```python
from build123d import *

# Parameters (mm, degrees)
SKETCH2_R           = 10.5
SKETCH2_R_2         = 7.5
BOSS_EXTRUDE1_DEPTH = 2.5
SKETCH2_3_R         = 7.5
SKETCH2_3_R_2       = 6.5
BOSS_EXTRUDE2_DEPTH = 1.5
SKETCH3_W           = 30
SKETCH3_H           = 6
CUT_EXTRUDE1_DEPTH  = 0.5
CUT_EXTRUDE2_START  = -1.5
CUT_EXTRUDE2_DEPTH  = 1.5
SKETCH5_R           = 5
SKETCH5_R_2         = 3.65
BOSS_EXTRUDE3_DEPTH = 1.5
FILLET1_R           = 0.5
CUT_EXTRUDE3_START  = -2.5
CUT_EXTRUDE3_DEPTH  = 2.5
BOSS_EXTRUDE4_DEPTH = 1.5
FILLET2_R           = 0.2


# Read off the part's stored shape, not the designer's step: Cut-Extrude3
with BuildPart() as part:
    # Sketch2 → Boss-Extrude1 (new body)
    with BuildSketch(Plane(origin=(0, 0, 0), x_dir=(1, 0, 0), z_dir=(0, 1, 0))):
        with Locations(Location((0, 0, 0), (0, 0, 270))):
            Circle(SKETCH2_R)
        with Locations(Location((0, 0, 0), (0, 0, 270))):
            Circle(SKETCH2_R_2, mode=Mode.SUBTRACT)
    extrude(amount=BOSS_EXTRUDE1_DEPTH)

    # Sketch2<3> → Boss-Extrude2 (add)
    with BuildSketch(Plane(origin=(0, 0, 0), x_dir=(1, 0, 0), z_dir=(0, 1, 0))):
        with Locations(Location((0, 0, 0), (0, 0, 270))):
            Circle(SKETCH2_3_R)
        with Locations(Location((0, 0, 0), (0, 0, 270))):
            Circle(SKETCH2_3_R_2, mode=Mode.SUBTRACT)
    extrude(amount=BOSS_EXTRUDE2_DEPTH)

    # Sketch3 → Cut-Extrude1 (cut)
    with BuildSketch(Plane(origin=(0, 2.5, 0), x_dir=(1, 0, 0), z_dir=(0, 1, 0))):
        Rectangle(SKETCH3_W, SKETCH3_H)
    extrude(amount=-CUT_EXTRUDE1_DEPTH, mode=Mode.SUBTRACT)

    # Sketch4 → Cut-Extrude2 (cut)
    with BuildSketch(Plane(origin=(0, 2.5, 0), x_dir=(1, 0, 0), z_dir=(0, 1, 0)).offset(CUT_EXTRUDE2_START)):
        with BuildLine():
            Line((-4, -9.708243919), (4, -9.708243919))
            ThreePointArc((4, -9.708243919), (0, -8.05), (-4, -9.708243919))
        make_face()
        with BuildLine():
            ThreePointArc((-4, -9.708243919), (0, -10.5), (4, -9.708243919))
            Line((4, -9.708243919), (-4, -9.708243919))
        make_face()
    extrude(amount=CUT_EXTRUDE2_DEPTH, mode=Mode.SUBTRACT)

    # Sketch5 → Boss-Extrude3 (add)
    # profile 1 of 6: a face of its own
    with BuildSketch(Plane(origin=(0, 0, 0), x_dir=(1, 0, 0), z_dir=(0, 1, 0))):
        Circle(SKETCH5_R)
        Circle(SKETCH5_R_2, mode=Mode.SUBTRACT)
    # profile 2 of 6: a face of its own
    with BuildSketch(Plane(origin=(0, 0, 0), x_dir=(1, 0, 0), z_dir=(0, 1, 0))):
        with BuildLine():
            Line((-4.307149461, -2.539382508), (-5.394288115, -3.626521162))
            ThreePointArc((-5.394288115, -3.626521162), (-4.596194078, -4.596194078), (-3.626521162, -5.394288115))
            Line((-3.626521162, -5.394288115), (-2.539382508, -4.307149461))
            ThreePointArc((-2.539382508, -4.307149461), (-3.535533906, -3.535533906), (-4.307149461, -2.539382508))
        make_face()
    # profile 3 of 6: a face of its own
    with BuildSketch(Plane(origin=(0, 0, 0), x_dir=(1, 0, 0), z_dir=(0, 1, 0))):
        with BuildLine():
            ThreePointArc((2.965697363, -2.127707487), (3.308023423, -1.542556655), (3.536232016, -0.904191975))
            Line((3.536232016, -0.904191975), (2.777613741, -0.550442464))
            Line((2.777613741, -0.550442464), (2.207079088, -1.773957976))
            Line((2.207079088, -1.773957976), (2.965697363, -2.127707487))
        make_face()
    # profile 4 of 6: a face of its own
    with BuildSketch(Plane(origin=(0, 0, 0), x_dir=(1, 0, 0), z_dir=(0, 1, 0))):
        with BuildLine():
            Line((-2.639832216, -1.02440757), (-3.325497417, -1.504515512))
            ThreePointArc((-3.325497417, -1.504515512), (-2.989904962, -2.093553993), (-2.551169228, -2.610370772))
            Line((-2.551169228, -2.610370772), (-1.865504027, -2.13026283))
            Line((-1.865504027, -2.13026283), (-2.639832216, -1.02440757))
        make_face()
    # profile 5 of 6: a face of its own
    with BuildSketch(Plane(origin=(0, 0, 0), x_dir=(1, 0, 0), z_dir=(0, 1, 0))):
        with BuildLine():
            Line((0.432753129, 2.798365546), (0.359800054, 3.632223))
            ThreePointArc((0.359800054, 3.632223), (-0.318118461, 3.636110648), (-0.985062788, 3.514562747))
            Line((-0.985062788, 3.514562747), (-0.912109714, 2.680705293))
            Line((-0.912109714, 2.680705293), (0.432753129, 2.798365546))
        make_face()
    # profile 6 of 6: a face of its own
    with BuildSketch(Plane(origin=(0, 0, 0), x_dir=(1, 0, 0), z_dir=(0, 1, 0))):
        with BuildLine():
            ThreePointArc((5.394288115, 3.626521162), (4.596194078, 4.596194078), (3.626521162, 5.394288115))
            Line((3.626521162, 5.394288115), (2.539382508, 4.307149461))
            ThreePointArc((2.539382508, 4.307149461), (3.535533906, 3.535533906), (4.307149461, 2.539382508))
            Line((4.307149461, 2.539382508), (5.394288115, 3.626521162))
        make_face()
    extrude(amount=BOSS_EXTRUDE3_DEPTH)

    # Fillet1
    fillet1_edges = [part.edges().sort_by_distance(p)[0] for p in [
        (5.394288115, 0.75, -3.626521162),
        (3.626521162, 0.75, -5.394288115),
        (-5.394288115, 0.75, 3.626521162),
        (-3.626521162, 0.75, 5.394288115),
    ]]
    fillet(fillet1_edges, radius=FILLET1_R)

    # Cut-Extrude3 outline → Cut-Extrude3 (cut)
    with BuildSketch(Plane(origin=(0, 2.5, 0), x_dir=(1, 0, 0), z_dir=(0, 1, 0)).offset(CUT_EXTRUDE3_START)):
        with BuildLine():
            Line((-1.104124308, 7.273205617), (-0.895875692, 6.437966041))
            ThreePointArc((-0.895875692, 6.437966041), (0, 6.5), (0.895875692, 6.437966041))
            Line((0.895875692, 6.437966041), (1.104124308, 7.273205617))
            ThreePointArc((1.104124308, 7.273205617), (0, 9.4), (-1.104124308, 7.273205617))
        make_face()
    extrude(amount=CUT_EXTRUDE3_DEPTH, mode=Mode.SUBTRACT)

    # Sketch7 → Boss-Extrude4 (add)
    with BuildSketch(Plane.XZ):
        with BuildLine():
            Line((1.05, 6.667886814), (1.9, 6.667886814))
            ThreePointArc((1.9, 6.667886814), (2.041421356, 6.726465457), (2.1, 6.867886814))
            Line((2.1, 6.867886814), (2.1, 9.467886814))
            ThreePointArc((2.1, 9.467886814), (2.041421356, 9.60930817), (1.9, 9.667886814))
            Line((1.9, 9.667886814), (1.05, 9.667886814))
            ThreePointArc((1.05, 9.667886814), (0.908578644, 9.60930817), (0.85, 9.467886814))
            Line((0.85, 9.467886814), (0.85, 6.867886814))
            ThreePointArc((0.85, 6.867886814), (0.908578644, 6.726465457), (1.05, 6.667886814))
        make_face()
        with BuildLine():
            Line((-2.1, 6.867886814), (-2.1, 9.467886814))
            ThreePointArc((-2.1, 9.467886814), (-2.041421356, 9.60930817), (-1.9, 9.667886814))
            Line((-1.9, 9.667886814), (-1.05, 9.667886814))
            ThreePointArc((-1.05, 9.667886814), (-0.908578644, 9.60930817), (-0.85, 9.467886814))
            Line((-0.85, 9.467886814), (-0.85, 6.867886814))
            ThreePointArc((-0.85, 6.867886814), (-0.908578644, 6.726465457), (-1.05, 6.667886814))
            Line((-1.05, 6.667886814), (-1.9, 6.667886814))
            ThreePointArc((-1.9, 6.667886814), (-2.041421356, 6.726465457), (-2.1, 6.867886814))
        make_face()
    extrude(amount=BOSS_EXTRUDE4_DEPTH)

    # Fillet2
    fillet2_edges = [part.edges().sort_by_distance(p)[0] for p in [
        (2.041421356, -1.5, 6.726465457),
        (2.1, -1.5, 8.167886814),
        (2.041421356, -1.5, 9.60930817),
        (1.475, -1.5, 9.667886814),
        (0.908578644, -1.5, 9.60930817),
        (0.85, -1.5, 8.167886814),
        (0.908578644, -1.5, 6.726465457),
        (1.475, -1.5, 6.667886814),
        (-0.908578644, -1.5, 9.60930817),
        (-1.475, -1.5, 9.667886814),
        (-2.041421356, -1.5, 9.60930817),
        (-2.1, -1.5, 8.167886814),
        (-2.041421356, -1.5, 6.726465457),
        (-1.475, -1.5, 6.667886814),
        (-0.908578644, -1.5, 6.726465457),
        (-0.85, -1.5, 8.167886814),
    ]]
    fillet(fillet2_edges, radius=FILLET2_R)


solid = part.part
```
Input: part model. Units: mm. Frame: model coordinates. A direction names the side the tool comes from. Give positions to 0.01 mm unless a question says otherwise; leave off trailing zeros. Order: outer loops, then holes, each group sorted by start corner. A loop starts at its lowest first (then second) coordinate and runs counter-clockwise, first axis right, second up.
1. Cut plane D-D (x = 0). Return loops of the section in (y, z), and give its area (3 significant figures).
Computed:
outline: (0, -10.5) - (2.5, -10.5) - (2.5, -9.4) - (0, -9.4) - close; (0, -5) - (1.5, -5) - (1.5, -2.76) - (0, -2.76) - close; (0, 3.65) - (1.5, 3.65) - (1.5, 5) - (0, 5) - close; (0, 6.5) - (1.5, 6.5) - (1.5, 7.5) - (2.5, 7.5) - (2.5, 8.05) - (1, 8.05) - (1, 10.5) - (0, 10.5) - close
area: 13.5 mm2
2. Cut plane C-C (z = -8.05). Return loops of the section in (x, y).
Computed:
outline: (-6.74, 0) - (-1.35, 0) - (-1.35, 2.5) - (-6.74, 2.5) - close; (1.35, 0) - (6.74, 0) - (6.74, 2.5) - (1.35, 2.5) - close
3. Pin query (flat end, axial travel): pin 1 Ø1.1 at (x, z) = (8.5, 0) entering from +Y; pin 2 Ø1.5 at (y, z) = (2, 8) entering from -X; pin 3 Ø0.9 at (x, y) = (-1.5, -0.5) entering from +Z. Return the tip coordinate at first contact, or that it passes through.
Computed:
pin 1: stops at y = 2
pin 2: stops at x = -7.6
pin 3: stops at z = 9.67
4. Set-up query: faces 5 (the face through (1.5, -0.6, 9.668)), 6 (the face through (-9, 2, 0)), 7 (the face through (-2.1, -1, 8)), 8 (the face through (3.2, 1.5, 1.6)), 9 (the face through (2.5, 0.74, 1.15)). Return all of +Z, -Z, +X, -X, +Y, -Y with unobstructed straight access to the full face (end or side cutting, diameter ignored); none if empty.
Computed:
face 5: +Z, +X, -X, -Y
face 6: +X, -X, +Y
face 7: +Z, -Z, -X, -Y
face 8: +Y
face 9: +Y, -Y
5. Cut plane B-B (y = -0.7). Return loops of the section in (x, z).
Computed:
outline: (-2.1, 6.87) arc R0.2 ccw to (-1.9, 6.67) - (-1.05, 6.67) arc R0.2 ccw to (-0.85, 6.87) - (-0.85, 9.47) arc R0.2 ccw to (-1.05, 9.67) - (-1.9, 9.67) arc R0.2 ccw to (-2.1, 9.47) - close; (0.85, 6.87) arc R0.2 ccw to (1.05, 6.67) - (1.9, 6.67) arc R0.2 ccw to (2.1, 6.87) - (2.1, 9.47) arc R0.2 ccw to (1.9, 9.67) - (1.05, 9.67) arc R0.2 ccw to (0.85, 9.47) - close
6. Draft query along Z for faces 1 (the face through (1, 0.74, -6.85)), 2 (the face through (1.5, -0.6, 6.668)), 3 (the face through (4.51, 0.74, 4.68)), 4 (the face through (-0.85, -1, 8)). Return one class per face: released by +Z, released by -Z, zero draft, split by the parting line, or undercut.
Computed:
face 1: undercut
face 2: released by -Z
face 3: undercut
face 4: zero draft
7. Line query: probe 1 along Z at (x, y) = (-2.25, 0.8); probe 2 along Y at (x, z) = (-8.5, 3.5); probe 3 along Y at (x, z) = (1.25, -4). Output: solid intervals per line, ascending.
Computed:
probe 1: z = -10.26 to -6.1, -4.47 to -2.87, 1.58 to 2.4, 2.87 to 4.47, 6.1 to 10.26
probe 2: y = 0 to 2.5
probe 3: y = 0 to 1.5
8. Cut plane A-A (z = 0). Return loops of the section in (x, y), and give its area (4 significant figures).
Computed:
outline: (-10.5, 0) - (-6.5, 0) - (-6.5, 1.5) - (-7.5, 1.5) - (-7.5, 2) - (-10.5, 2) - close; (-5, 0) - (-3.65, 0) - (-3.65, 1.5) - (-5, 1.5) - close; (3.65, 0) - (5, 0) - (5, 1.5) - (3.65, 1.5) - close; (6.5, 0) - (10.5, 0) - (10.5, 2) - (7.5, 2) - (7.5, 1.5) - (6.5, 1.5) - close
area: 19.05 mm2
